Work out the finished part from the listing and answer in its coordinate system (mm). A direction names the side the tool comes from. Round coordinates to 2 decimals unless told otherwise and drop trailing zeros. Order: outer loops, then holes, each group sorted by start corner. A loop starts at its lowest first (then second) coordinate and runs counter-clockwise, first axis right, second up. Notation, with made-up numbers: (37, 89) - (45, 89) arc R17 cw to (45, 96) - close; hole circle Ø3 at (-12, -28). An arc over 180 degrees is marked (long way). Use one line per item in the form item = value. Start each with the question number.
Q1. The part is cut by section C-C on z = 23.5. Determine the outline of the cut face in (x, y), plus the area to 3 significant figures.
Q2. The part is cut by section B-B on x = 54. Determine the outline of the cut face in (y, z).
Q3. The part is cut by section D-D on x = 27. Determine the outline of the cut face in (y, z), plus the area to 3 significant figures.
Q4. For a pull along X with two mould halves and no side action, classify faces 1 (the flat face through (33.537, 4.437, 41.693)), 2 (the flat face through (29, -18, 9)), 3 (the cylindrical face through (18.246, -22.348, 4.437)) as +X half, -X half, draft (parallel to the pull), parting line (faces both ways), or undercut.
Q5. Find the intervals of material crossed by line 1 (Y direction, x = 46, z = 3); line 2 (Z direction, x = 54, y = -14); line 3 (X direction, y = -27, z = 4.5), in increasing order. Write a range as [from, to].
Q6. The part is cut by section A-A on y = -4.5. Determine the outline of the cut face in (x, z).
Q7. Given P1, Ø11, axis at x = 36.5, y = -13, coming from the +Z side; P2, Ø4.5, axis at y = -17.5, z = 6, coming from the +X side; P3, Ø22.5, axis at x = 24.5, z = 38.5, coming from the -Y side; P4, Ø8, axis at x = 45, z = 61.5, coming from the -Y side, each flat-ended and moving along its own axis, determine where each tip first touches the part or whether it passes through.
Q8. Which of the six approach directions +Z, -Z, +X, -X, +Y, -Y give full straight-line access (tool end or side, diameter ignored) to faces 4 (the flat face through (59, -12, 4)), 5 (the flat face through (76.67, -13.82, 66.67)), 6 (the flat face through (75.048, 4.437, 26.712))?
from build123d import *

# Parameters (mm, degrees)
F0_R     = 5.5
F1_DEPTH = 9
F2_W     = 59
F2_H     = 9
F3_DEPTH = 9
F4_R     = 7
F4_W     = 9
F4_H     = 32
F5_DEPTH = 9


with BuildPart() as f1:
    # F0 (on Top) → F1 (new body)
    with BuildSketch(Plane.XY):
        with BuildLine():
            Line((59, 0), (0, 0))
            Line((0, 0), (0, -24))
            ThreePointArc((0, -24), (3.807612, -33.192388), (13, -37))
            Line((13, -37), (46, -37))
            ThreePointArc((46, -37), (55.192388, -33.192388), (59, -24))
            Line((59, -24), (59, 0))
        make_face()
        with Locations((13, -24)):
            Circle(F0_R, mode=Mode.SUBTRACT)
        with Locations((46, -24)):
            Circle(F0_R, mode=Mode.SUBTRACT)
    extrude(amount=F1_DEPTH)

    # F2 (on face) → F3 (join)
    with BuildSketch(Plane(origin=(0, 0, 0), x_dir=(-1, 0, 0), z_dir=(0, 1, 0))):
        Polygon((-90.653089, 52.686292), (-59, 0), (-59, 9), (0, 9), (-68.025672, 75.313708), align=None)
        with Locations((-29.5, 4.5)):
            Rectangle(F2_W, F2_H)
    extrude(amount=F3_DEPTH)

    # F4 (on face) → F5 (join)
    with BuildSketch(Plane(origin=(71.66969, 0, 71.66969), x_dir=(0, 1, 0), z_dir=(0.707107, 0, 0.707107))):
        with BuildLine():
            Line((0, -26.84658), (0, 5.15342))
            Line((0, 5.15342), (-20, 5.15342))
            ThreePointArc((-20, 5.15342), (-36, -10.84658), (-20, -26.84658))
            Line((-20, -26.84658), (0, -26.84658))
        make_face()
        with Locations((-20, -10.84658)):
            Circle(F4_R, mode=Mode.SUBTRACT)
        with Locations((4.5, -10.84658)):
            Rectangle(F4_W, F4_H)
    extrude(amount=F5_DEPTH)


solid = f1.part
Found:
q1.outline = (14.87, 0) - (73.12, 0) - (73.12, 9) - (14.87, 9) - close
q1.area = 524 mm²
q2.outline = (-34.25, 0) - (9, 0) - (9, 61.64) - (0, 61.64) - (0, 9) - (-34.25, 9) - close
q3.outline = (-37, 0) - (9, 0) - (9, 35.32) - (0, 35.32) - (0, 9) - (-37, 9) - close
q3.area = 651 mm²
q4.face_1 = -X half
q4.face_2 = draft
q4.face_3 = undercut
q5.line_1 = [-37, -29.5], [-18.5, 9]
q5.line_2 = [0, 9]
q5.line_3 = [0.35, 8.39], [17.61, 41.39], [50.61, 58.65]
q6.outline = (0, 0) - (59, 0) - (59, 9) - (0, 9) - close; (68.03, 75.31) - (90.65, 52.69) - (97.02, 59.05) - (74.39, 81.68) - close
q7.P1 = 9
q7.P2 = 59
q7.P3 = 0
q7.P4 = through
q8.face_4 = +Z, -Z, +X, -Y
q8.face_5 = -Z, -X, -Y
q8.face_6 = -Z, +X, +Y, -Y
